Job drawing, mm, ordinate dimensions from the low corner. One solid piece. Round coordinates to 2 decimals unless told otherwise and drop trailing zeros. Write each loop counter-clockwise with the first axis right and the second up, starting at its lowest first coordinate (ties: lowest second). Pieces come first, ordered by that corner, then holes.
1) Drill centre lines: L1, parallel to Z at x = 15.5, y = 1.4; L2, parallel to X at y = 3.25, z = 28; L3, parallel to Z at x = 3.25, y = 2.45. Where is each one in solid material? Low to high.
2) Saw through at C-C on y = 3.1. Write the cut outline in (x, z), and give its area (3 significant figures).
3) Saw through at B-B on z = 13. Write the cut outline in (x, y), and give its area (3 significant figures).
4) Flat gauge pin, fed straight in: pin 1 (2.5 mm diameter, centred on x = 15.5, z = 13, fed in from -Y). Where does the tip first touch, or does it go through?
5) Saw through at A-A on x = 2.5. Write the cut outline in (y, z), and give its area (3 significant figures).
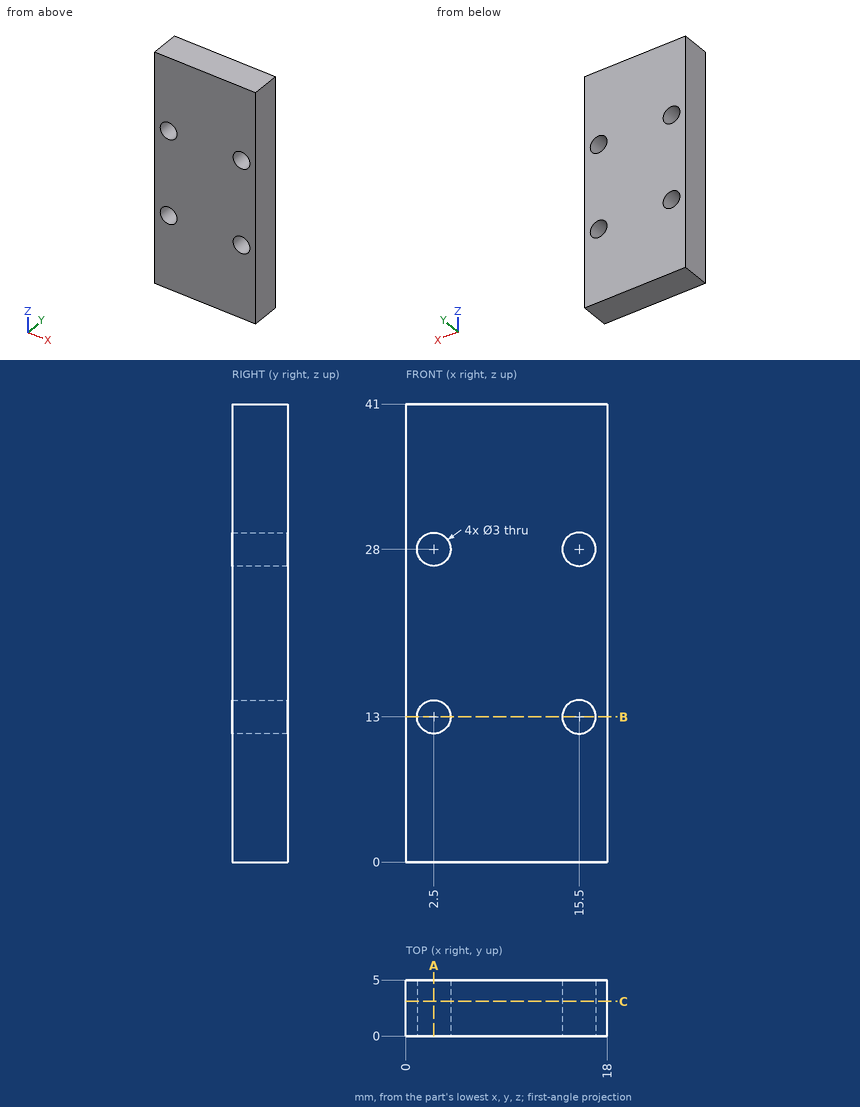
Completed:
1. L1: z = 0 to 11.5, 14.5 to 26.5, 29.5 to 41
1. L2: x = 0 to 1, 4 to 14, 17 to 18
1. L3: z = 0 to 11.7, 14.3 to 26.7, 29.3 to 41
2. outline: (0, 0) - (18, 0) - (18, 41) - (0, 41) - close; hole circle Ø3 at (2.5, 13); hole circle Ø3 at (2.5, 28); hole circle Ø3 at (15.5, 13); hole circle Ø3 at (15.5, 28)
2. area: 710 mm2
3. outline: (0, 0) - (1, 0) - (1, 5) - (0, 5) - close; (4, 0) - (14, 0) - (14, 5) - (4, 5) - close; (17, 0) - (18, 0) - (18, 5) - (17, 5) - close
3. area: 60.0 mm2
4. pin 1: passes through
5. outline: (0, 0) - (5, 0) - (5, 11.5) - (0, 11.5) - close; (0, 14.5) - (5, 14.5) - (5, 26.5) - (0, 26.5) - close; (0, 29.5) - (5, 29.5) - (5, 41) - (0, 41) - close
5. area: 175 mm2
